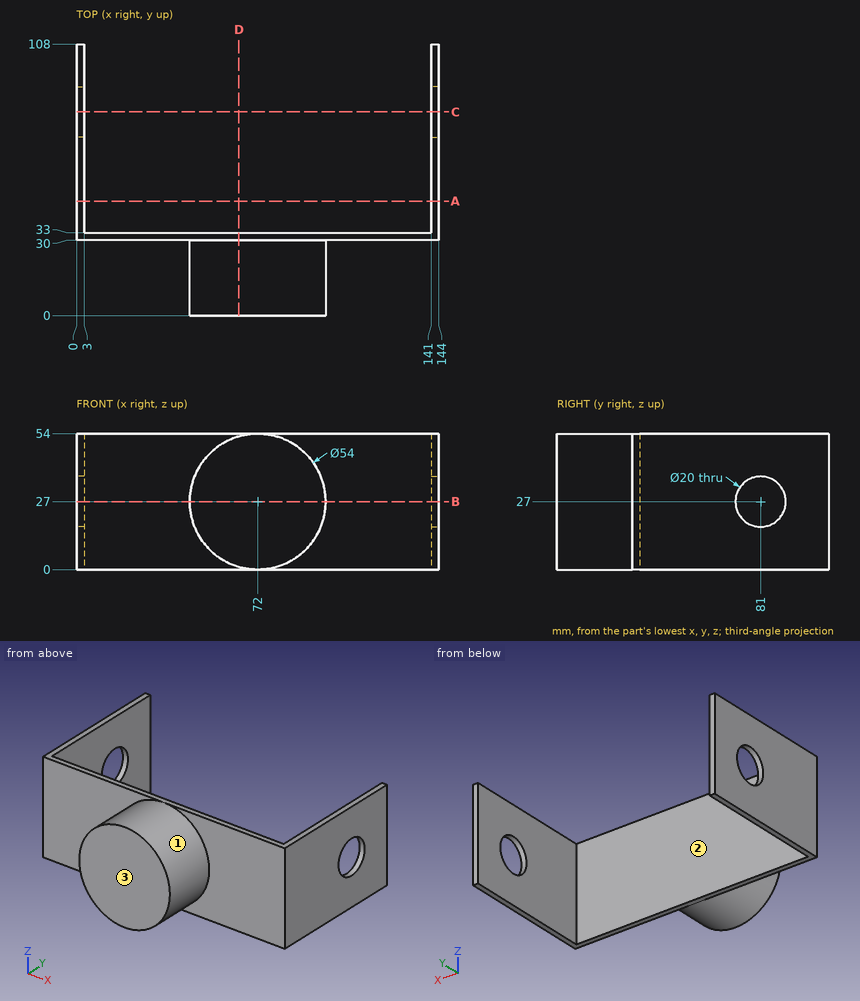
Verification items for this drawing (mm, ordinates from the low corner). A direction names the side the tool comes from. Coordinates: 2 decimals unless noted, no trailing zeros. Loops run counter-clockwise (first coordinate to the right, second up) from the corner with the lowest first, then second, coordinate; pieces in that order, holes last. Notation, with made-up numbers: (1.5, 9.25) - (47.5, 9.25) arc R22 ccw to (47.5, 20.25) - close; hole circle Ø4 at (-38.75, 13.25). An arc over 180 degrees is marked (long way). One line per item, written item: value. Start each with the question number.
(1) Cross-section at D-D on x = 64.5. Enter the section's corners in (y, z).
(2) Cross-section at A-A on y = 45.5. Enter the section's corners in (x, z), plus the area to 3 significant figures.
(3) Cross-section at C-C on y = 81. Enter the section's corners in (x, z).
(4) Cross-section at B-B on z = 27. Enter the section's corners in (x, y), plus the area to 3 significant figures.
(5) Material ranges on line 1 (X direction, y = 68, z = 49); line 2 (Z direction, x = 1.5, y = 81); line 3 (Y direction, x = 31, z = 12), recorded low to high. Write a range as [from, to].
(6) Tool access check on the marked faces 1, 2 and 3. Record the directions out of +Z, -Z, +X, -X, +Y, -Y that give a thin tool (end or side, any length) a straight path to the whole face; none if there is none.
(7) Depth check by flat-ended pin: P1, Ø1, axis at x = 54, z = 28, coming from the +Y side; P2, Ø1.5, axis at y = 20, z = 29, coming from the +X side. Enter the tip coordinate at first touch or a pass-through.
Results below:
1. outline: (0, 1.06) - (30, 1.06) - (30, 0) - (33, 0) - (33, 54) - (30, 54) - (30, 52.94) - (0, 52.94) - close
2. outline: (0, 0) - (3, 0) - (3, 54) - (0, 54) - close; (141, 0) - (144, 0) - (144, 54) - (141, 54) - close
2. area: 324 mm2
3. outline: (0, 0) - (3, 0) - (3, 17) - (0, 17) - close; (0, 37) - (3, 37) - (3, 54) - (0, 54) - close; (141, 0) - (144, 0) - (144, 17) - (141, 17) - close; (141, 37) - (144, 37) - (144, 54) - (141, 54) - close
4. outline: (0, 30) - (45, 30) - (45, 0) - (99, 0) - (99, 30) - (144, 30) - (144, 71) - (141, 71) - (141, 33) - (3, 33) - (3, 71) - (0, 71) - close; (0, 91) - (3, 91) - (3, 108) - (0, 108) - close; (141, 91) - (144, 91) - (144, 108) - (141, 108) - close
4. area: 2,380 mm2
5. line 1: x = [0, 3], [141, 144]
5. line 2: z = [0, 17], [37, 54]
5. line 3: y = [30, 33]
6. face 1: -Y
6. face 2: +Z, -Z, +Y
6. face 3: +Z, -Z, +X, -X, -Y
7. P1: stops at y = 33
7. P2: stops at x = 98.97
